```python
from build123d import *

# Parameters (mm, degrees)
ESQUISSE4_W             = 130
ESQUISSE4_H             = 100
BOSS_EXTRU_4_DEPTH      = 55
CONG_5_R                = 20
ENL_V_MAT_EXTRU_1_DEPTH = 47
CONG_6_SIZE             = 10


with BuildPart() as part:
    # Esquisse4 → Boss.-Extru.4 (new body)
    with BuildSketch(Plane(origin=(0, 0, 0), x_dir=(1, 0, 0), z_dir=(0, 1, 0))):
        with Locations((12.771948074, 16.229726537)):
            Rectangle(ESQUISSE4_W, ESQUISSE4_H)
    extrude(amount=BOSS_EXTRU_4_DEPTH)

    # Congé5
    cong_5_edges = [part.edges().sort_by_distance(p)[0] for p in [
        (-52.228051926, 27.5, -66.229726537),
        (77.771948074, 27.5, -66.229726537),
        (77.771948074, 27.5, 33.770273463),
        (-52.228051926, 27.5, 33.770273463),
    ]]
    fillet(cong_5_edges, radius=CONG_5_R)

    # Esquisse5 → Enlèv. mat.-Extru.1 (cut)
    with BuildSketch(Plane(origin=(0, 55, 0), x_dir=(1, 0, 0), z_dir=(0, 1, 0))):
        with BuildLine():
            Line((57.771948074, 58.229726537), (-32.228051926, 58.229726537))
            ThreePointArc((-32.228051926, 58.229726537), (-40.713333301, 54.715007912), (-44.228051926, 46.229726537))
            Line((-44.228051926, 46.229726537), (-44.228051926, -13.770273463))
            ThreePointArc((-44.228051926, -13.770273463), (-40.713333301, -22.255554837), (-32.228051926, -25.770273463))
            Line((-32.228051926, -25.770273463), (57.771948074, -25.770273463))
            ThreePointArc((57.771948074, -25.770273463), (66.257229448, -22.255554837), (69.771948074, -13.770273463))
            Line((69.771948074, -13.770273463), (69.771948074, 46.229726537))
            ThreePointArc((69.771948074, 46.229726537), (66.257229448, 54.715007912), (57.771948074, 58.229726537))
        make_face()
    extrude(amount=-ENL_V_MAT_EXTRU_1_DEPTH, mode=Mode.SUBTRACT)

    # Congé6
    # a fillet whose section is not a circle: 10 mm, written as the material it adds along each edge
    with BuildSketch(Plane(origin=(57.771948074, 8, -46.229726537), x_dir=(1, 0, 0), z_dir=(0, 0, 1))) as cong_6_piece_1:
        with BuildLine():
            Bezier((12, CONG_6_SIZE), (12, 0), (12 - CONG_6_SIZE, 0), weights=[1, 0.707106781, 1])
            Line((12 - CONG_6_SIZE, 0), (12, 0))
            Line((12, 0), (12, CONG_6_SIZE))
        make_face()
    revolve(axis=Axis((57.771948074, 8, -46.229726537), (0, 1, 0)), revolution_arc=90)
    with BuildSketch(Plane(origin=(69.771948074, 8, 13.770273463), x_dir=(0, 1, 0), z_dir=(0, 0, -1)), Plane(origin=(-44.228051926, 8, -46.229726537), x_dir=(0, 1, 0), z_dir=(0, 0, 1))) as cong_6_piece_2:
        with BuildLine():
            Bezier((CONG_6_SIZE, 0), (0, 0), (0, -CONG_6_SIZE), weights=[1, 0.707106781, 1])
            Line((0, -CONG_6_SIZE), (0, 0))
            Line((0, 0), (CONG_6_SIZE, 0))
        make_face()
    extrude(amount=60)
    with BuildSketch(Plane(origin=(57.771948074, 8, 13.770273463), x_dir=(0, 0, 1), z_dir=(-1, 0, 0))) as cong_6_piece_3:
        with BuildLine():
            Bezier((12, CONG_6_SIZE), (12, 0), (12 - CONG_6_SIZE, 0), weights=[1, 0.707106781, 1])
            Line((12 - CONG_6_SIZE, 0), (12, 0))
            Line((12, 0), (12, CONG_6_SIZE))
        make_face()
    revolve(axis=Axis((57.771948074, 8, 13.770273463), (0, 1, 0)), revolution_arc=90)
    with BuildSketch(Plane(origin=(-32.228051926, 8, 25.770273463), x_dir=(0, 1, 0), z_dir=(1, 0, 0)), Plane(origin=(57.771948074, 8, -58.229726537), x_dir=(0, 1, 0), z_dir=(-1, 0, 0))) as cong_6_piece_4:
        with BuildLine():
            Bezier((CONG_6_SIZE, 0), (0, 0), (0, -CONG_6_SIZE), weights=[1, 0.707106781, 1])
            Line((0, -CONG_6_SIZE), (0, 0))
            Line((0, 0), (CONG_6_SIZE, 0))
        make_face()
    extrude(amount=90)
    with BuildSketch(Plane(origin=(-32.228051926, 8, 13.770273463), x_dir=(-1, 0, 0), z_dir=(0, 0, -1))) as cong_6_piece_5:
        with BuildLine():
            Bezier((12, CONG_6_SIZE), (12, 0), (12 - CONG_6_SIZE, 0), weights=[1, 0.707106781, 1])
            Line((12 - CONG_6_SIZE, 0), (12, 0))
            Line((12, 0), (12, CONG_6_SIZE))
        make_face()
    revolve(axis=Axis((-32.228051926, 8, 13.770273463), (0, 1, 0)), revolution_arc=90)
    with BuildSketch(Plane(origin=(-32.228051926, 8, -46.229726537), x_dir=(0, 0, -1), z_dir=(1, 0, 0))) as cong_6_piece_6:
        with BuildLine():
            Bezier((12, CONG_6_SIZE), (12, 0), (12 - CONG_6_SIZE, 0), weights=[1, 0.707106781, 1])
            Line((12 - CONG_6_SIZE, 0), (12, 0))
            Line((12, 0), (12, CONG_6_SIZE))
        make_face()
    revolve(axis=Axis((-32.228051926, 8, -46.229726537), (0, 1, 0)), revolution_arc=90)


solid = part.part
```
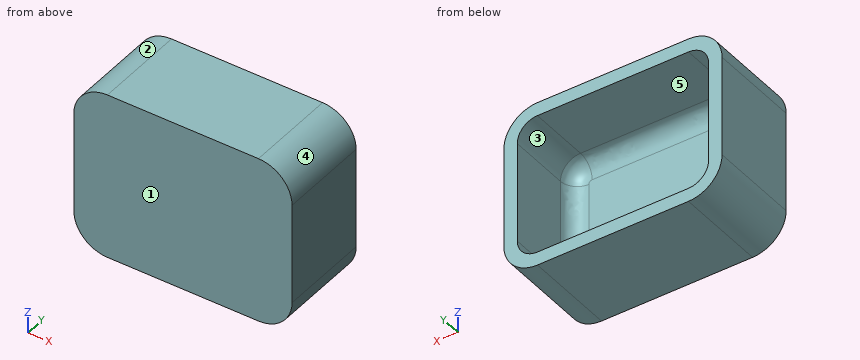
Read the model definition and answer for the solid it produces. Units are mm, in the model's axes. Face numbers are marked on the shaded views. A direction names the side the tool comes from. Round coordinates to 2 decimals unless told otherwise and drop trailing zeros. Write each loop counter-clockwise with the first axis right and the second up, starting at its lowest first coordinate (ties: lowest second). Pieces come first, ordered by that corner, then holes. Notation, with made-up numbers: (-6.5, 77.5) -> (16.5, 77.5) arc R19 ccw to (16.5, 102.5) -> close; hole circle Ø7 at (68.25, 64). An arc over 180 degrees is marked (long way). Answer in a Markdown table with one row per item. Add a question column.
1) Find section B-B, the plane y = 6. Determine the outline of the cut face in (x, z).
2) Consider line 1 (X direction, y = 22, z = -14); line 2 (Z direction, x = -18, y = 20.5); line 3 (X direction, y = 29, z = 22). Determine where each line is inside the solid, lowest interval first.
3) Determine the mould class of the marked faces 1, 2 and 3 for opening direction Z: pulls with the +Z half, pulls with the -Z half, needs draft (parallel to the pull), parting line crosses it, or undercut.
4) Find section A-A, the plane y = 28. Determine the outline of the cut face in (x, z), and give its area (3 significant figures).
5) Which of the six approach directions +Z, -Z, +X, -X, +Y, -Y give full straight-line access (tool end or side, diameter ignored) to the marked faces 4 and 5?
6) Given P1, Ø1.5, axis at y = 17.5, z = -53.5, coming from the -X side, flat-ended and moving along its own axis, determine where the tip first touches the part or whether it passes through.
Findings below:
| question | item | result |
|---|---|---|
| 1 | outline | (-52.23, -46.23) arc R20 ccw to (-32.23, -66.23) -> (57.77, -66.23) arc R20 ccw to (77.77, -46.23) -> (77.77, 13.77) arc R20 ccw to (57.77, 33.77) -> (-32.23, 33.77) arc R20 ccw to (-52.23, 13.77) -> close |
| 2 | line 1 | -52.23 to -44.23, 69.77 to 77.77 |
| 2 | line 2 | -66.23 to -58.23, 25.77 to 33.77 |
| 2 | line 3 | -50.46 to -40.96, 66.51 to 76 |
| 3 | face 1 | needs draft |
| 3 | face 2 | pulls with the +Z half |
| 3 | face 3 | undercut |
| 4 | outline | (-52.23, -46.23) arc R20 ccw to (-32.23, -66.23) -> (57.77, -66.23) arc R20 ccw to (77.77, -46.23) -> (77.77, 13.77) arc R20 ccw to (57.77, 33.77) -> (-32.23, 33.77) arc R20 ccw to (-52.23, 13.77) -> close; hole (-44.23, -46.23) arc R12 ccw to (-32.23, -58.23) -> (57.77, -58.23) arc R12 ccw to (69.77, -46.23) -> (69.77, 13.77) arc R12 ccw to (57.77, 25.77) -> (-32.23, 25.77) arc R12 ccw to (-44.23, 13.77) -> close |
| 4 | area | 3,200 mm² |
| 5 | face 4 | +Z, +X, +Y, -Y |
| 5 | face 5 | +Y |
| 6 | P1 | x = -51.14 |
